Geometry: final body of the model. Coordinates: model frame, mm. A direction names the side the tool comes from. Give positions to 0.01 mm unless a question says otherwise; leave off trailing zeros. Loops run counter-clockwise (first coordinate to the right, second up) from the corner with the lowest first, then second, coordinate; pieces in that order, holes last.
1. First-contact query: P1, Ø2, axis at y = 1.5, z = -1, coming from the -X side (3 decimals). Flat tip, straight axial feed; report the tip coordinate or a pass-through.
2. Draft query along Z for faces 1 (the face through (0, 11, 0)), 2 (the face through (1, 10, -1)), 3 (the face through (0.25, 4.93, 1.15)). Return one class per face: +Z half, -Z half, draft (parallel to the pull), parting line (faces both ways), or undercut.
3. Section A-A, the plane z = -0.9. Output: boundary loops of the cut face in (x, y), then the cut area to 3 significant figures.
4. Material intervals for line 1 along Y through (x, z) = (-0.85, -0.9); line 2 along Y through (x, z) = (0.05, -0.35); line 3 along X through (y, z) = (6.5, 0.8), sorted ascending.
5. Access query for faces 4 (the face through (0.071, 11.507, 0.747)), 5 (the face through (0, 0, 0)). Directions: +Z, -Z, +X, -X, +Y, -Y. A direction counts if a zero-diameter tool reaches every point of the face in a straight line with its end or side. Return the directions, or none.
6. Section C-C, the plane y = 5.5. Output: boundary loops of the cut face in (x, z) (3 decimals).
7. Section B-B, the plane x = -0.05. Output: boundary loops of the cut face in (y, z).
8. Section D-D, the plane z = -0.35. Output: boundary loops of the cut face in (x, y).
Autodesk Inventor part; units mm, degrees
ref_plane "YZ Plane" through (0, 0, 0) normal (1, 0, 0) x (0, 1, 0)
ref_plane "XZ Plane" through (0, 0, 0) normal (0, 1, 0) x (-1, 0, 0)
ref_plane "XY Plane" through (0, 0, 0) normal (0, 0, 1) x (1, 0, 0)
sketch "Sketch1" plane through (0, 0, 0) normal (0, 1, 0) x (-1, 0, 0)
  circle A0 centre (0, 0) radius 1.175
  dimension "d0" = 2.35
extrude "Extrusion1" add sketch "Sketch1" along normal blind 10
sketch "Sketch2" plane through (0, 10, 0) normal (0, 1, 0) x (1, 0, 0)
  circle A0 centre (0, 0) radius 1.175
  circle A1 centre (0, 0) radius 1.925
  dimension "d3" = 3.85
extrude "Extrusion2" add sketch "Sketch2" along normal blind 2 contours A0 | A1
sketch "Sketch3" plane through (0, 12, 0) normal (0, 1, 0) x (1, 0, 0)
  line L0 (-0.4961, 0.7099) -> (0.3667, 0.7845)
  line L1 (0.3667, 0.7845) -> (0.8628, 0.0747)
  line L2 (0.8628, 0.0747) -> (0.4961, -0.7099)
  line L3 (0.4961, -0.7099) -> (-0.3667, -0.7845)
  line L4 (-0.3667, -0.7845) -> (-0.8628, -0.0747)
  line L5 (-0.8628, -0.0747) -> (-0.4961, 0.7099)
  point P0 (0, 0)
  point P1 (0, 0)
  dimension "d6" = 1.5
extrude "Extrusion3" cut sketch "Sketch3" against normal blind 1
equation "\"d0\" = M2_A"
equation "\"d3\" = M2_B"
properties part number "M2_SCREW_8MM"
Answers below:
1. P1: stops at x = -1.175
2. face 1: undercut
2. face 2: draft
2. face 3: parting line
3. outline: (-1.7, 10) - (-0.76, 10) - (-0.76, 0) - (0.76, 0) - (0.76, 10) - (1.7, 10) - (1.7, 12) - (-1.7, 12) - close
3. area: 21.9 mm2
4. line 1: y = 10 to 12
4. line 2: y = 0 to 11
4. line 3: x = -0.86 to 0.86
5. face 4: +Y
5. face 5: +Z, -Z, +X, -X, -Y
6. outline: circle Ø2.35 at (0, 0)
7. outline: (0, -1.17) - (10, -1.17) - (10, -1.92) - (12, -1.92) - (12, -0.75) - (11, -0.75) - (11, 0.76) - (12, 0.76) - (12, 1.92) - (10, 1.92) - (10, 1.17) - (0, 1.17) - close
8. outline: (-1.89, 10) - (-1.12, 10) - (-1.12, 0) - (1.12, 0) - (1.12, 10) - (1.89, 10) - (1.89, 12) - (0.67, 12) - (0.67, 11) - (-0.66, 11) - (-0.66, 12) - (-1.89, 12) - close
